Source: three-view drawing plus pictorial views. Frame: mm from the lowest corner of the part. A direction names the side the tool comes from. Give positions to 0.01 mm unless a question says otherwise; leave off trailing zeros. Loops run counter-clockwise (first coordinate to the right, second up) from the corner with the lowest first, then second, coordinate; pieces in that order, holes last. Notation, with made-up numbers: (85.25, -12.5) - (118.25, -12.5) arc R10 cw to (118.25, 1.5) - close; hole circle Ø2 at (11.25, 15). An arc over 180 degrees is marked (long way). One line per item, written item: value.
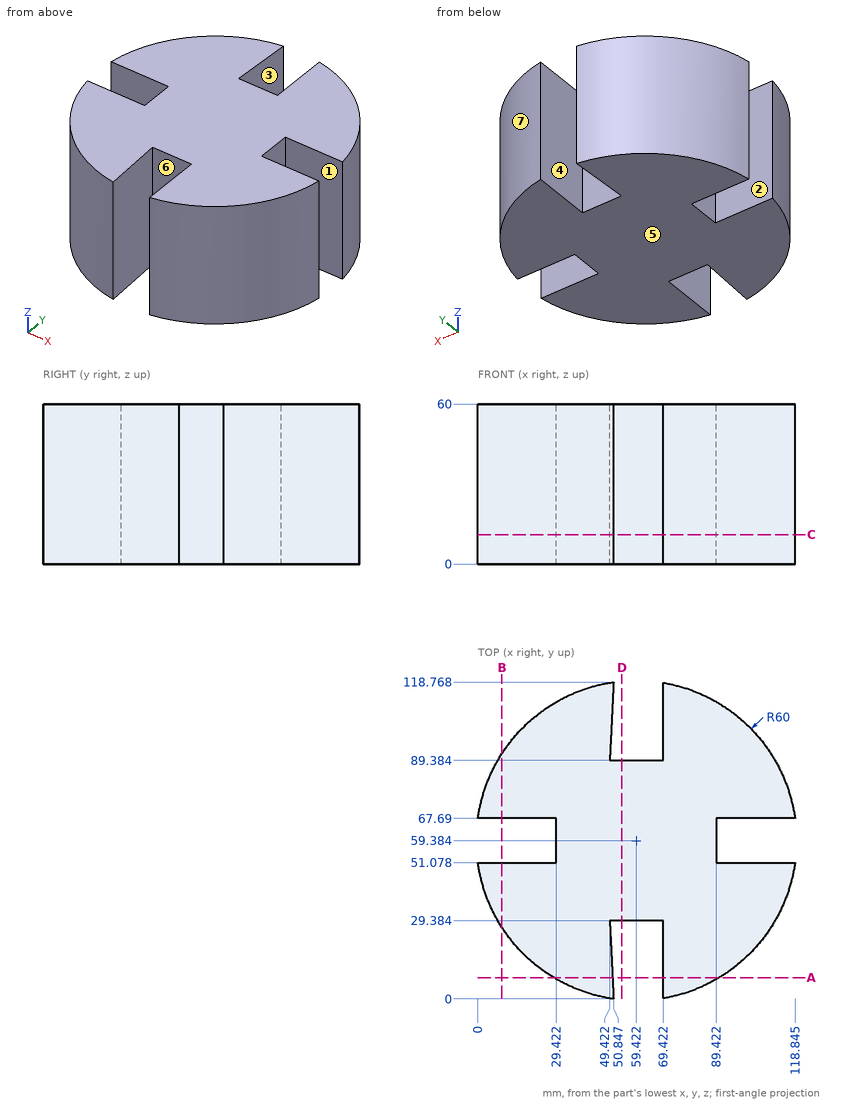
Item 1: Pin query (flat end, axial travel): P1, Ø9, axis at x = 13.5, z = 38.5, coming from the -Y side; P2, Ø12, axis at y = 19.5, z = 35, coming from the -X side (1 decimal); P3, Ø14.5, axis at x = 102.5, z = 44, coming from the +Y side. Return the tip coordinate at first contact, or that it passes through.
Verdict:
P1: stops at y = 15.98
P2: stops at x = 9.9
P3: stops at y = 107.51
Item 2: Access query for the marked faces 1, 2 and 3. Directions: +Z, -Z, +X, -X, +Y, -Y. A direction counts if a zero-diameter tool reaches every point of the face in a straight line with its end or side. Return the directions, or none.
Verdict:
face 1: +Z, -Z, +X
face 2: +Z, -Z, -X
face 3: +Z, -Z
Item 3: Draft query along X for the marked faces 4, 5, 6 and 7. Return one class per face: pulls with the +X half, pulls with the -X half, needs draft (parallel to the pull), parting line crosses it, or undercut.
Verdict:
face 4: undercut
face 5: needs draft
face 6: undercut
face 7: pulls with the +X half
Item 4: Material intervals for L1, parallel to X at y = 59, z = 54; L2, parallel to Y at x = 93.5, z = 54.5; L3, parallel to Y at x = 66, z = 46, sorted ascending.
Verdict:
L1: x = 29.42 to 89.42
L2: y = 10 to 51.08, 67.69 to 108.77
L3: y = 29.38 to 89.38
Item 5: Section C-C, the plane z = 11. Output: boundary loops of the cut face in (x, y) (1 decimal), and give its area (3 significant figures).
Verdict:
outline: (0, 51.1) arc R60 ccw to (50.8, 0) - (49.4, 29.4) - (69.4, 29.4) - (69.4, 0.2) arc R60 ccw to (118.8, 51.1) - (89.4, 51.1) - (89.4, 67.7) - (118.8, 67.7) arc R60 ccw to (69.4, 118.5) - (69.4, 89.4) - (49.4, 89.4) - (50.8, 118.8) arc R60 ccw to (0, 67.7) - (29.4, 67.7) - (29.4, 51.1) - close
area: 9,170 mm^2
Item 6: Section D-D, the plane x = 54. Output: boundary loops of the cut face in (y, z), and give its area (3 significant figures).
Verdict:
outline: (29.38, 0) - (89.38, 0) - (89.38, 60) - (29.38, 60) - close
area: 3,600 mm^2
Item 7: Section A-A, the plane y = 8. Output: boundary loops of the cut face in (x, z).
Verdict:
outline: (28.44, 0) - (50.46, 0) - (50.46, 60) - (28.44, 60) - close; (69.42, 0) - (90.4, 0) - (90.4, 60) - (69.42, 60) - close
Item 8: Section B-B, the plane x = 9. Output: boundary loops of the cut face in (y, z) (1 decimal).
Verdict:
outline: (26.9, 0) - (51.1, 0) - (51.1, 60) - (26.9, 60) - close; (67.7, 0) - (91.9, 0) - (91.9, 60) - (67.7, 60) - close
